from build123d import *

# Parameters (mm, degrees)
SKETCH_W        = 240
SKETCH_H        = 20
PAD_DEPTH       = 200
SKETCH001_W     = 200
SKETCH001_H     = 180
POCKET_DEPTH    = 20.001
SKETCH002_W     = 100
SKETCH002_H     = 10
PAD001_DEPTH    = 30
SKETCH003_R     = 2.5
HOLE_DEPTH      = 0.497848
HOLE_TIPS_R     = 2.5
SKETCH004_W     = 10
SKETCH004_H     = 6
POCKET001_DEPTH = 7.5
SKETCH005_W     = 10
SKETCH005_H     = 5
POCKET002_DEPTH = 15
SKETCH006_W     = 20
SKETCH006_H     = 30
PAD002_DEPTH    = 30
CHAMFER_SIZE    = 24
SKETCH007_W     = 110
SKETCH007_H     = 50
PAD003_DEPTH    = 20
FILLET_R        = 3
FILLET_FACE8_W  = 104
FILLET_FACE8_H  = 44
POCKET003_DEPTH = 10
CHAMFER001_SIZE = 10


with BuildPart() as part:
    # Sketch → Pad (new body)
    with BuildSketch(Plane.XY):
        Rectangle(SKETCH_W, SKETCH_H)
    extrude(amount=PAD_DEPTH)

    # Sketch001 (on Face3 of Pad) → Pocket (cut, through all)
    with BuildSketch(Plane.XZ.offset(10)):
        with Locations((0, 90)):
            Rectangle(SKETCH001_W, SKETCH001_H)
    extrude(amount=-POCKET_DEPTH, mode=Mode.SUBTRACT)

    # Sketch002 (on Face4 of Pocket) → Pad001 (join)
    with BuildSketch(Plane(origin=(0, 0, 180), x_dir=(1, 0, 0), z_dir=(0, 0, -1))):
        Rectangle(SKETCH002_W, SKETCH002_H)
    extrude(amount=PAD001_DEPTH)

    # Sketch003 (on Face14 of Pad001) → Hole (cut)
    with BuildSketch(Plane.XZ.offset(5)):
        with Locations((-40, 170)):
            Circle(SKETCH003_R)
        with Locations((-20, 170)):
            Circle(SKETCH003_R)
        with Locations((0, 170)):
            Circle(SKETCH003_R)
        with Locations((20, 170)):
            Circle(SKETCH003_R)
        with Locations((40, 170)):
            Circle(SKETCH003_R)
        with Locations((-40, 160)):
            Circle(SKETCH003_R)
        with Locations((-20, 160)):
            Circle(SKETCH003_R)
        with Locations((0, 160)):
            Circle(SKETCH003_R)
        with Locations((20, 160)):
            Circle(SKETCH003_R)
        with Locations((40, 160)):
            Circle(SKETCH003_R)
    extrude(amount=-HOLE_DEPTH, mode=Mode.SUBTRACT)

    # Hole tips → Hole tip 1 section 0
    with BuildSketch(Plane.XZ.offset(4.502152), mode=Mode.PRIVATE) as hole_tip_1_s0:
        with Locations((-40, 170)):
            Circle(HOLE_TIPS_R)
    loft([hole_tip_1_s0.sketch, Vertex(-40, -3, 170)], mode=Mode.SUBTRACT)

    # Hole tips → Hole tip 2 section 0
    with BuildSketch(Plane.XZ.offset(4.502152), mode=Mode.PRIVATE) as hole_tip_2_s0:
        with Locations((-20, 170)):
            Circle(HOLE_TIPS_R)
    loft([hole_tip_2_s0.sketch, Vertex(-20, -3, 170)], mode=Mode.SUBTRACT)

    # Hole tips → Hole tip 3 section 0
    with BuildSketch(Plane.XZ.offset(4.502152), mode=Mode.PRIVATE) as hole_tip_3_s0:
        with Locations((0, 170)):
            Circle(HOLE_TIPS_R)
    loft([hole_tip_3_s0.sketch, Vertex(0, -3, 170)], mode=Mode.SUBTRACT)

    # Hole tips → Hole tip 4 section 0
    with BuildSketch(Plane.XZ.offset(4.502152), mode=Mode.PRIVATE) as hole_tip_4_s0:
        with Locations((20, 170)):
            Circle(HOLE_TIPS_R)
    loft([hole_tip_4_s0.sketch, Vertex(20, -3, 170)], mode=Mode.SUBTRACT)

    # Hole tips → Hole tip 5 section 0
    with BuildSketch(Plane.XZ.offset(4.502152), mode=Mode.PRIVATE) as hole_tip_5_s0:
        with Locations((40, 170)):
            Circle(HOLE_TIPS_R)
    loft([hole_tip_5_s0.sketch, Vertex(40, -3, 170)], mode=Mode.SUBTRACT)

    # Hole tips → Hole tip 6 section 0
    with BuildSketch(Plane.XZ.offset(4.502152), mode=Mode.PRIVATE) as hole_tip_6_s0:
        with Locations((-40, 160)):
            Circle(HOLE_TIPS_R)
    loft([hole_tip_6_s0.sketch, Vertex(-40, -3, 160)], mode=Mode.SUBTRACT)

    # Hole tips → Hole tip 7 section 0
    with BuildSketch(Plane.XZ.offset(4.502152), mode=Mode.PRIVATE) as hole_tip_7_s0:
        with Locations((-20, 160)):
            Circle(HOLE_TIPS_R)
    loft([hole_tip_7_s0.sketch, Vertex(-20, -3, 160)], mode=Mode.SUBTRACT)

    # Hole tips → Hole tip 8 section 0
    with BuildSketch(Plane.XZ.offset(4.502152), mode=Mode.PRIVATE) as hole_tip_8_s0:
        with Locations((0, 160)):
            Circle(HOLE_TIPS_R)
    loft([hole_tip_8_s0.sketch, Vertex(0, -3, 160)], mode=Mode.SUBTRACT)

    # Hole tips → Hole tip 9 section 0
    with BuildSketch(Plane.XZ.offset(4.502152), mode=Mode.PRIVATE) as hole_tip_9_s0:
        with Locations((20, 160)):
            Circle(HOLE_TIPS_R)
    loft([hole_tip_9_s0.sketch, Vertex(20, -3, 160)], mode=Mode.SUBTRACT)

    # Hole tips → Hole tip 10 section 0
    with BuildSketch(Plane.XZ.offset(4.502152), mode=Mode.PRIVATE) as hole_tip_10_s0:
        with Locations((40, 160)):
            Circle(HOLE_TIPS_R)
    loft([hole_tip_10_s0.sketch, Vertex(40, -3, 160)], mode=Mode.SUBTRACT)

    # Sketch004 (on Face3 of Hole) → Pocket001 (cut, symmetric)
    with BuildSketch(Plane.YZ.offset(-100)):
        with Locations((0, 15)):
            Rectangle(SKETCH004_W, SKETCH004_H)
    extrude(amount=POCKET001_DEPTH, both=True, mode=Mode.SUBTRACT)

    # Sketch005 (on Face5 of Pocket001) → Pocket002 (cut)
    with BuildSketch(Plane(origin=(100, 0, 0), x_dir=(0, -1, 0), z_dir=(-1, 0, 0))):
        with Locations((0, 14.5)):
            Rectangle(SKETCH005_W, SKETCH005_H)
    extrude(amount=-POCKET002_DEPTH, mode=Mode.SUBTRACT)

    # Sketch006 (on Face7 of Pocket002) → Pad002 (join)
    with BuildSketch(Plane.YZ.offset(120)):
        with Locations((0, 15)):
            Rectangle(SKETCH006_W, SKETCH006_H)
    extrude(amount=PAD002_DEPTH)

    # Chamfer
    chamfer_edges = [part.edges().sort_by_distance(p)[0] for p in [
        (150, 0, 30),
    ]]
    chamfer(chamfer_edges, length=CHAMFER_SIZE)

    # Sketch007 (on Face3 of Chamfer) → Pad003 (join)
    with BuildSketch(Plane(origin=(78, 0, 78), x_dir=(0, 1, 0), z_dir=(0.707107, 0, 0.707107))):
        with Locations((0, -85.882251)):
            Rectangle(SKETCH007_W, SKETCH007_H)
    extrude(amount=PAD003_DEPTH)

    # Fillet
    fillet_edges = [part.edges().sort_by_distance(p)[0] for p in [
        (152.870058, -55, 31.414214),
        (170.547727, 0, 13.736544),
        (135.192388, 0, 49.091883),
        (152.870058, 55, 31.414214),
    ]]
    fillet(fillet_edges, radius=FILLET_R)

    # Fillet Face8 → Pocket003 (cut)
    with BuildSketch(Plane(origin=(152.870058, 0, 31.414214), x_dir=(0, -1, 0), z_dir=(0.707107, 0, 0.707107))):
        Rectangle(FILLET_FACE8_W, FILLET_FACE8_H)
    extrude(amount=-POCKET003_DEPTH, mode=Mode.SUBTRACT)

    # Chamfer001
    chamfer001_edges = [part.edges().sort_by_distance(p)[0] for p in [
        (120, 0, 200),
        (-120, 0, 200),
    ]]
    chamfer(chamfer001_edges, length=CHAMFER001_SIZE)


solid = part.part
Design review of the part built by this model. Coordinates are the model's own, in mm. A direction names the side the tool comes from. Round coordinates to 2 decimals unless told otherwise and drop trailing zeros. Write each loop counter-clockwise with the first axis right and the second up, starting at its lowest first coordinate (ties: lowest second). Pieces come first, ordered by that corner, then holes.
Item 1: For faces 4 (the flat face through (-2, 0, 200)), 5 (the flat face through (107, 0, 17)), 6 (the flat face through (-1, -7, 180)), 7 (the flat face through (-110, 0, 0)), list the 3-axis set-ups (+Z, -Z, +X, -X, +Y, -Y) from which the entire face can be reached by the end or side of a thin tool; tool diameter is ignored.
Item 2: Wall thickness on L1, parallel to Z at x = 0, y = -4.8; L2, parallel to Z at x = 0, y = -4; L3, parallel to X at y = 6.5, z = 77: over which ranges is each line inside the solid? List them lowest first.
Item 3: Consider section C-C on x = -34. Give the boundary of the cut face in (y, z), and give its area (3 significant figures).
Item 4: Draft analysis for pull direction Z (two halves, no side actions). For faces 1 (the flat face through (-100, 0, 89)), 2 (the flat face through (164.94, 0.73, 12.37)), 3 (the flat face through (133.828, 0.728, 43.485)), state which applies: released by +Z, released by -Z, zero draft, split by the parting line, or undercut.
Item 5: Consider section D-D on z = 184. Give the boundary of the cut face in (x, y), and give its area (3 significant figures).
Item 6: Consider section A-A on y = -14. Give the boundary of the cut face in (x, z).
Item 7: For pin 1 Ø22 at (x, y) = (-112, 2.5) entering from -Z; pin 2 Ø5.5 at (x, z) = (105.5, 15.5) entering from +Y; pin 3 Ø4 at (x, z) = (-20, 160) entering from -Y, all flat-tipped, find the tip position at first contact; note any pin that passes through.
Item 8: Consider section B-B on z = 136. Give the boundary of the cut face in (x, y), and give its area (3 significant figures).
Check values:
1. face 4: +Z, +X, -X, +Y, -Y
1. face 5: none
1. face 6: -Z
1. face 7: -Z, -X, +Y, -Y
2. L1: z = 150 to 157.5, 162.5 to 167.5, 172.5 to 200
2. L2: z = 150 to 158.34, 161.66 to 168.34, 171.66 to 200
2. L3: x = -120 to -100, 100 to 120
3. outline: (-10, 180) - (-5, 180) - (-5, 150) - (5, 150) - (5, 180) - (10, 180) - (10, 200) - (-10, 200) - close
3. area: 700 mm2
4. face 1: zero draft
4. face 2: released by +Z
4. face 3: undercut
5. outline: (-120, -10) - (120, -10) - (120, 10) - (-120, 10) - close
5. area: 4,800 mm2
6. outline: (121.05, 34.95) - (156.41, -0.41) - (168.43, 11.62) arc R3 ccw to (168.43, 15.86) - (161.36, 8.79) - (130.24, 39.9) - (137.31, 46.97) arc R3 ccw to (133.07, 46.97) - close
7. pin 1: stops at z = 0
7. pin 2: stops at y = 10
7. pin 3: stops at y = -4.2
8. outline: (-120, -10) - (-100, -10) - (-100, 10) - (-120, 10) - close; (100, -10) - (120, -10) - (120, 10) - (100, 10) - close
8. area: 800 mm2
